```python
from build123d import *

# Parameters (mm, degrees)
SKETCH1_W                        = 24
SKETCH1_H                        = 66
BOSS_EXTRUDE1_DEPTH              = 10
F_8_0MM_DOWEL_HOLE1_D            = 8
F_8_0MM_DOWEL_HOLE1_DEPTH        = 24.5
F_8_0MM_DOWEL_HOLE1_CSINK_D      = 8.05
F_8_0MM_DOWEL_HOLE1_CSINK_ANGLE  = 90
F_8_0MM_DOWEL_HOLE1_TIP          = 2.403442476
F_10_0MM_DOWEL_HOLE2_D           = 10
F_10_0MM_DOWEL_HOLE2_DEPTH       = 24.5
F_10_0MM_DOWEL_HOLE2_CSINK_D     = 10.05
F_10_0MM_DOWEL_HOLE2_CSINK_ANGLE = 90
F_10_0MM_DOWEL_HOLE2_TIP         = 3.004303095
FILLET1_R                        = 3


with BuildPart() as part:
    # Sketch1 → Boss-Extrude1 (new, symmetric)
    with BuildSketch(Plane.XY):
        Polygon((-18, -31.849478444), (-18, 31.849478444), (-12, 39), (12, 39), (18, 31.849478444), (18, -31.849478444), (12, -39), (-12, -39), align=None)
        Rectangle(SKETCH1_W, SKETCH1_H, mode=Mode.SUBTRACT)
    extrude(amount=BOSS_EXTRUDE1_DEPTH, both=True)

    # Ø8.0mm Dowel Hole1
    with Locations(Plane.ZX.offset(39)):
        with Locations((0, 0)):
            CounterSinkHole(F_8_0MM_DOWEL_HOLE1_D / 2, F_8_0MM_DOWEL_HOLE1_CSINK_D / 2, depth=F_8_0MM_DOWEL_HOLE1_DEPTH, counter_sink_angle=F_8_0MM_DOWEL_HOLE1_CSINK_ANGLE)
            with Locations((0, 0, -(F_8_0MM_DOWEL_HOLE1_DEPTH + F_8_0MM_DOWEL_HOLE1_TIP / 2))):  # 118° drill point
                Cone(0, F_8_0MM_DOWEL_HOLE1_D / 2, F_8_0MM_DOWEL_HOLE1_TIP, mode=Mode.SUBTRACT)

    # Ø10.0mm Dowel Hole2
    with Locations(Plane(origin=(0, -39, 0), x_dir=(0, 0, -1), z_dir=(0, -1, 0))):
        with Locations((0, 0)):
            CounterSinkHole(F_10_0MM_DOWEL_HOLE2_D / 2, F_10_0MM_DOWEL_HOLE2_CSINK_D / 2, depth=F_10_0MM_DOWEL_HOLE2_DEPTH, counter_sink_angle=F_10_0MM_DOWEL_HOLE2_CSINK_ANGLE)
            with Locations((0, 0, -(F_10_0MM_DOWEL_HOLE2_DEPTH + F_10_0MM_DOWEL_HOLE2_TIP / 2))):  # 118° drill point
                Cone(0, F_10_0MM_DOWEL_HOLE2_D / 2, F_10_0MM_DOWEL_HOLE2_TIP, mode=Mode.SUBTRACT)

    # Fillet1
    fillet1_edges = [part.edges().sort_by_distance(p)[0] for p in [
        (12, -33, 0),
        (12, 33, 0),
        (-12, 33, 0),
        (-12, -33, 0),
    ]]
    fillet(fillet1_edges, radius=FILLET1_R)


solid = part.part
```
Build history of the part. All positions in model axes, mm. A direction names the side the tool comes from. Round coordinates to 2 decimals unless told otherwise and drop trailing zeros. Write each loop counter-clockwise with the first axis right and the second up, starting at its lowest first coordinate (ties: lowest second). Pieces come first, ordered by that corner, then holes. Notation, with made-up numbers: (14.25, 67.5) - (42.25, 67.5) arc R29 cw to (42.25, 95.5) - close; hole circle Ø7 at (83.5, 24). An arc over 180 degrees is marked (long way). Write each question's results on one line, items separated by ' | '. Start each with the question number.
Item 1: Saw through at B-B (x = -6). Write the cut outline in (y, z).
Item 2: Saw through at D-D (x = 0). Write the cut outline in (y, z) (3 decimals).
Item 3: Mould opens along X. For faces 1 (the face through (18, 0, 0)), 2 (the face through (-14.96, -35.47, 0.14)), 3 (the face through (-12, 0, 0)) say: pulls with the +X half, pulls with the -X half, needs draft (parallel to the pull), parting line crosses it, or undercut.
Item 4: Drop a flat-ended pin along its axis: P1, Ø10, axis at x = 0, z = 1.5, coming from the +Y side. Give the stop position or say it passes through.
Item 5: Saw through at A-A (z = 0). Write the cut outline in (x, y) (3 decimals).
Item 6: Wall check: L1, parallel to X at y = -16.5, z = -5; L2, parallel to Y at x = 8, z = -7.25; L3, parallel to Z at x = 0, y = 36. Give the ranges that are in metal, low to high. Write a range as [from, to].
Item 7: Which spindle directions (+Z, -Z, +X, -X, +Y, -Y) get a long thin tool onto all of the face, cutting with end or side? Do faces 4 (the face through (0, 33, 5)), 5 (the face through (-4.88, -35.95, -1.08)), 6 (the face through (12.3, 0.5, 10)). Say none if no direction does.
Item 8: Saw through at C-C (y = 27.5). Write the cut outline in (x, z).
Results are:
1) outline: (-39, -10) - (-33, -10) - (-33, 10) - (-39, 10) - close; (33, -10) - (39, -10) - (39, 10) - (33, 10) - close
2) outline: (-39, -10) - (-33, -10) - (-33, -5) - (-38.975, -5) - (-39, -5.025) - close; (-39, 5.025) - (-38.975, 5) - (-33, 5) - (-33, 10) - (-39, 10) - close; (33, -10) - (39, -10) - (39, -4.025) - (38.975, -4) - (33, -4) - close; (33, 4) - (38.975, 4) - (39, 4.025) - (39, 10) - (33, 10) - close
3) face 1: pulls with the +X half | face 2: pulls with the -X half | face 3: undercut
4) P1: stops at y = 39
5) outline: (-18, -31.849) - (-12, -39) - (-5.025, -39) - (-5, -38.975) - (-5, -33) - (-9, -33) arc R3 cw to (-12, -30) - (-12, 30) arc R3 cw to (-9, 33) - (-4, 33) - (-4, 38.975) - (-4.025, 39) - (-12, 39) - (-18, 31.849) - close; (4, 33) - (9, 33) arc R3 cw to (12, 30) - (12, -30) arc R3 cw to (9, -33) - (5, -33) - (5, -38.975) - (5.025, -39) - (12, -39) - (18, -31.849) - (18, 31.849) - (12, 39) - (4.025, 39) - (4, 38.975) - close
6) L1: x = [-18, -12], [12, 18] | L2: y = [-39, -33], [33, 39] | L3: z = [-10, -4], [4, 10]
7) face 4: +Z, -Z | face 5: -Y | face 6: +Z, +X, -X, +Y, -Y
8) outline: (-18, -10) - (-12, -10) - (-12, 10) - (-18, 10) - close; (12, -10) - (18, -10) - (18, 10) - (12, 10) - close
